from build123d import *

# Parameters (mm, degrees)
PAD_DEPTH       = 63.5
SKETCH001_W     = 51.05
SKETCH001_H     = 51.05
POCKET_DEPTH    = 88.9
SKETCH002_W     = 51.05
SKETCH002_H     = 51.05
POCKET001_DEPTH = 88.9
SKETCH003_R     = 7.9375
PAD001_DEPTH    = 12.7
SKETCH004_R     = 2
POCKET002_DEPTH = 6.35
SKETCH005_R     = 2
POCKET003_DEPTH = 6.35
SKETCH006_W     = 81.05
SKETCH006_H     = 81.05
SKETCH006_W_2   = 51.05
SKETCH006_H_2   = 51.05
PAD002_DEPTH    = 10
SKETCH007_W     = 81.05
SKETCH007_H     = 81.05
SKETCH007_W_2   = 51.05
SKETCH007_H_2   = 51.05
PAD003_DEPTH    = 10
FILLET_R        = 1


with BuildPart() as part:
    # Sketch → Pad (new body)
    with BuildSketch(Plane.XZ):
        Polygon((0, 152.4), (0, 0), (152.4, 0), (152.4, 63.5), (63.5, 63.5), (63.5, 152.4), align=None)
    extrude(amount=PAD_DEPTH)

    # Sketch001 (on Face6 of Pad) → Pocket (cut)
    with BuildSketch(Plane(origin=(0, 0, 152.4), x_dir=(-1, 0, 0), z_dir=(0, 0, 1))):
        with Locations((-31.875, 31.875)):
            Rectangle(SKETCH001_W, SKETCH001_H)
    extrude(amount=-POCKET_DEPTH, mode=Mode.SUBTRACT)

    # Sketch002 (on Face11 of Pocket) → Pocket001 (cut)
    with BuildSketch(Plane(origin=(152.4, 0, 0), x_dir=(0, 0, 1), z_dir=(1, 0, 0))):
        with Locations((31.875, 31.875)):
            Rectangle(SKETCH002_W, SKETCH002_H)
    extrude(amount=-POCKET001_DEPTH, mode=Mode.SUBTRACT)

    # Sketch003 → Pad001 (join)
    with BuildSketch(Plane.XZ.offset(25.4)):
        Polygon((63.5, 152.4), (63.5, 63.5), (152.4, 63.5), align=None)
        with Locations((90.979437, 90.979437)):
            Circle(SKETCH003_R, mode=Mode.SUBTRACT)
    extrude(amount=PAD001_DEPTH)

    # Sketch004 (on Face1 of Pad001) → Pocket002 (cut)
    with BuildSketch(Plane(origin=(0, 0, 0), x_dir=(0, 0, -1), z_dir=(-1, 0, 0))):
        with Locations((-130, 31.75)):
            Circle(SKETCH004_R)
        with Locations((-88.9, 31.75)):
            Circle(SKETCH004_R)
    extrude(amount=-POCKET002_DEPTH, mode=Mode.SUBTRACT)

    # Sketch005 (on Face5 of Pocket002) → Pocket003 (cut)
    with BuildSketch(Plane(origin=(0, 0, 0), x_dir=(1, 0, 0), z_dir=(0, 0, -1))):
        with Locations((88.9, 31.75)):
            Circle(SKETCH005_R)
        with Locations((130, 31.75)):
            Circle(SKETCH005_R)
    extrude(amount=-POCKET003_DEPTH, mode=Mode.SUBTRACT)

    # Sketch006 (on Face2 of Pocket003) → Pad002 (join)
    with BuildSketch(Plane(origin=(0, 0, 152.4), x_dir=(-1, 0, 0), z_dir=(0, 0, 1))):
        with Locations((-31.875, 31.875)):
            Rectangle(SKETCH006_W, SKETCH006_H)
        with Locations((-31.875, 31.875)):
            Rectangle(SKETCH006_W_2, SKETCH006_H_2, mode=Mode.SUBTRACT)
    extrude(amount=-PAD002_DEPTH)

    # Sketch007 (on Face18 of Pad002) → Pad003 (join)
    with BuildSketch(Plane(origin=(152.4, 0, 0), x_dir=(0, 0, 1), z_dir=(1, 0, 0))):
        with Locations((31.875, 31.875)):
            Rectangle(SKETCH007_W, SKETCH007_H)
        with Locations((31.875, 31.875)):
            Rectangle(SKETCH007_W_2, SKETCH007_H_2, mode=Mode.SUBTRACT)
    extrude(amount=-PAD003_DEPTH)

    # Fillet
    fillet_edges = [part.edges().sort_by_distance(p)[0] for p in [
        (63.5, -50.8, 63.5),
        (63.5, -12.7, 63.5),
        (63.5, -50.8, 142.4),
        (63.5, -12.7, 142.4),
        (142.4, -50.8, 63.5),
        (142.4, -12.7, 63.5),
        (142.4, -25.4, 67.95),
        (142.4, -38.1, 67.95),
        (67.95, -38.1, 142.4),
        (67.95, -25.4, 142.4),
        (102.95, -25.4, 63.5),
        (63.5, -25.4, 102.95),
        (102.95, 0, 63.5),
        (63.5, 0, 102.95),
        (72.4, -25.4, 142.95),
        (72.4, 8.65, 147.4),
        (147.4, 8.65, 72.4),
        (147.4, 8.65, -8.65),
        (147.4, -72.4, -8.65),
        (142.4, -31.75, 0),
        (142.4, 0, 31.75),
        (31.75, 0, 142.4),
        (147.4, -72.4, 72.4),
        (-8.65, 8.65, 147.4),
        (-8.65, -72.4, 147.4),
        (72.4, -72.4, 147.4),
        (-8.65, -31.875, 142.4),
        (31.875, 8.65, 142.4),
        (0, -31.75, 142.4),
        (31.75, -63.5, 142.4),
        (31.875, -72.4, 142.4),
        (0, -63.5, 71.2),
        (71.2, -63.5, 0),
        (0, -31.75, 0),
        (0, 0, 71.2),
        (71.2, 0, 0),
        (142.4, 8.65, 31.875),
        (142.4, -31.875, -8.65),
        (31.875, 8.65, 152.4),
        (-8.65, -31.875, 152.4),
        (31.875, -72.4, 152.4),
        (72.4, -31.875, 152.4),
        (152.4, -72.4, 31.875),
        (152.4, -31.875, -8.65),
        (152.4, 8.65, 31.875),
        (152.4, -31.875, 72.4),
        (102.95, -63.5, 63.5),
        (63.5, -63.5, 102.95),
        (142.4, -72.4, 31.875),
        (142.95, -38.1, 72.4),
        (142.95, -25.4, 72.4),
        (72.4, -38.1, 142.95),
    ]]
    fillet(fillet_edges, radius=FILLET_R)


solid = part.part
CAD build for the part. Positions are in the model's coordinates, mm. A direction names the side the tool comes from. Round coordinates to 2 decimals unless told otherwise and drop trailing zeros. Order: outer loops, then holes, each group sorted by start corner. A loop starts at its lowest first (then second) coordinate and runs counter-clockwise, first axis right, second up. Notation, with made-up numbers: (69.25, -23) - (95.25, -23) arc R25 ccw to (95.25, -11) - close; hole circle Ø9 at (4.25, 19). An arc over 180 degrees is marked (long way). Return JSON: item names as keys, results as strings.
(1) Pull direction X, two halves, no side cores. Call faces 1 (the face through (-8.65, -31, 147)), 2 (the face through (103, -25.4, 95)), 3 (the face through (55, -63.5, 57)): +X half, -X half, draft (parallel to the pull), parting line (faces both ways), or undercut.
Answer key:
{"face 1": "-X half", "face 2": "undercut", "face 3": "draft"}
(2) Cut at C-C (x = 88.9). Give the cut face in (y, z), then the cut area to 3 significant figures.
Answer key:
{"outline": "(-63.5, 1) arc R1 ccw to (-62.5, 0) - (-33.75, 0) - (-33.75, 6.35) - (-57.4, 6.35) - (-57.4, 57.4) - (-6.35, 57.4) - (-6.35, 6.35) - (-29.75, 6.35) - (-29.75, 0) - (-1, 0) arc R1 ccw to (0, 1) - (0, 62.5) arc R1 ccw to (-1, 63.5) - (-24.4, 63.5) arc R1 cw to (-25.4, 64.5) - (-25.4, 83.32) - (-38.1, 83.32) - (-38.1, 63.5) - (-62.5, 63.5) arc R1 ccw to (-63.5, 62.5) - close; (-38.1, 98.64) - (-25.4, 98.64) - (-25.4, 127) - (-38.1, 127) - close", "area": "2,010 mm^2"}
(3) Cut at D-D (x = 130). Give the cut face in (y, z), then the cut area to 3 significant figures.
Answer key:
{"outline": "(-63.5, 1) arc R1 ccw to (-62.5, 0) - (-33.75, 0) - (-33.75, 6.35) - (-57.4, 6.35) - (-57.4, 57.4) - (-6.35, 57.4) - (-6.35, 6.35) - (-29.75, 6.35) - (-29.75, 0) - (-1, 0) arc R1 ccw to (0, 1) - (0, 62.5) arc R1 ccw to (-1, 63.5) - (-24.4, 63.5) arc R1 cw to (-25.4, 64.5) - (-25.4, 85.9) - (-38.1, 85.9) - (-38.1, 63.5) - (-62.5, 63.5) arc R1 ccw to (-63.5, 62.5) - close", "area": "1,680 mm^2"}
(4) Cut at B-B (z = 108.5). Give the cut face in (x, y), then the cut area to 3 significant figures.
Answer key:
{"outline": "(0, -62.5) arc R1 ccw to (1, -63.5) - (62.5, -63.5) arc R1 ccw to (63.5, -62.5) - (63.5, -38.1) - (107.4, -38.1) - (107.4, -25.4) - (64.5, -25.4) arc R1 cw to (63.5, -24.4) - (63.5, -1) arc R1 ccw to (62.5, 0) - (1, 0) arc R1 ccw to (0, -1) - close; hole (6.35, -57.4) - (57.4, -57.4) - (57.4, -6.35) - (6.35, -6.35) - close", "area": "1,980 mm^2"}
(5) Wall check: probe 1 along Z at (x, y) = (1.5, -31.75); probe 2 along Y at (x, z) = (2.5, 130). Give the ranges that are in metal, low to high. Write a range as from..to.
Answer key:
{"probe 1": "z = 0..86.9, 90.9..128, 132..152.4", "probe 2": "y = -63.5..-33.75, -29.75..0"}
(6) Cut at A-A (y = -67). Give the cut face in (x, z), then the cut area to 3 significant figures.
Answer key:
{"outline": "(-8.65, 143.4) arc R1 ccw to (-7.65, 142.4) - (72.4, 142.4) - (72.4, 151.4) arc R1 ccw to (71.4, 152.4) - (-7.65, 152.4) arc R1 ccw to (-8.65, 151.4) - close; (142.4, -7.65) arc R1 ccw to (143.4, -8.65) - (151.4, -8.65) arc R1 ccw to (152.4, -7.65) - (152.4, 71.4) arc R1 ccw to (151.4, 72.4) - (142.4, 72.4) - close", "area": "1,620 mm^2"}
(7) Pin check, flat tips, straight feed: pin 1 Ø2 at (x, z) = (82, 86) entering from -Y; pin 2 Ø4 at (y, z) = (-2, 86.5) entering from -X; pin 3 Ø15.5 at (x, z) = (34, 111.5) entering from -Y. Stop position of each tip, or through.
Answer key:
{"pin 1": "stops at y = -38.1", "pin 2": "stops at x = 0", "pin 3": "stops at y = -63.5"}
(8) Tool access for faces 4 (the face through (109, -57.4, 32)), 5 (the face through (55, 0, 57)), 6 (the face through (32, -6.35, 109)), 7 (the face through (-3, -32, 142.4)): list every direction of +Z, -Z, +X, -X, +Y, -Y with a clear straight run to the whole face (end or side of a thin tool).
Answer key:
{"face 4": "+X", "face 5": "-Z, -X, +Y", "face 6": "+Z", "face 7": "none"}
